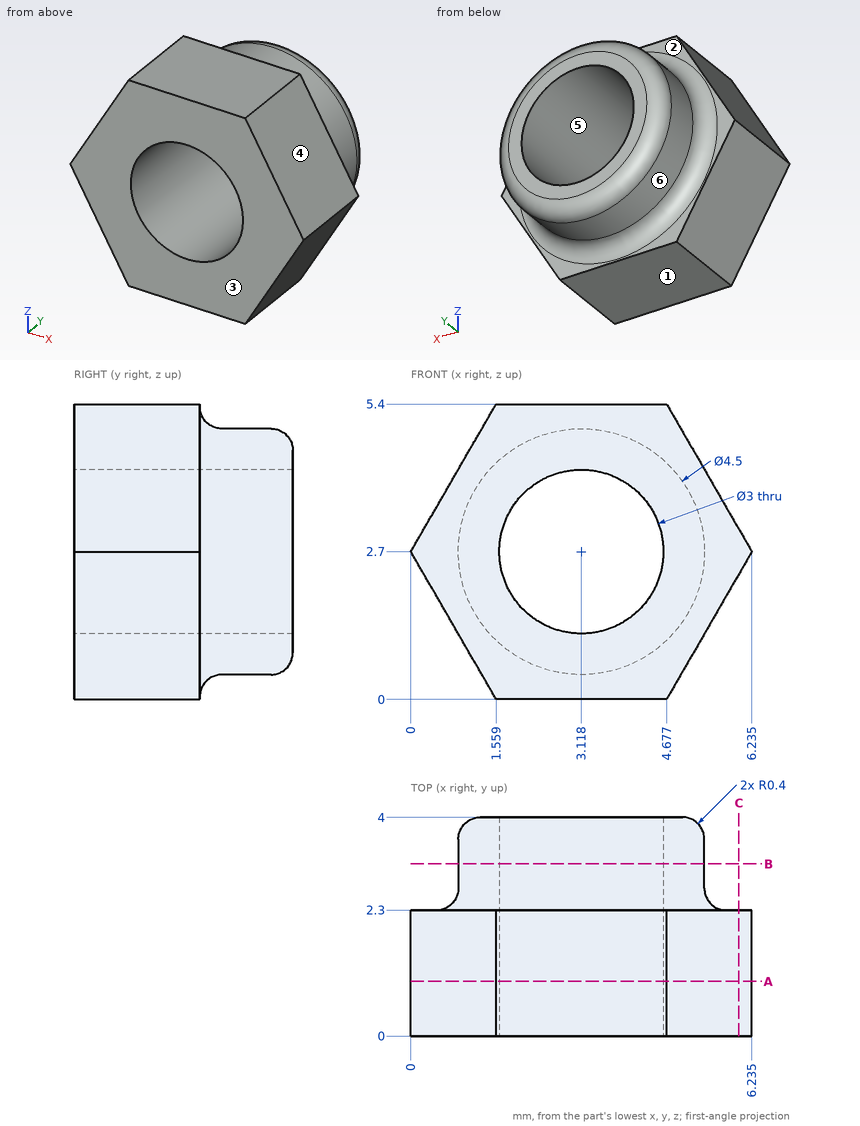
Geometry check sheet. Reference: drawing and pictorial views, mm from the part's lowest x, y, z. A direction names the side the tool comes from. Round coordinates to 2 decimals unless told otherwise and drop trailing zeros. Loops run counter-clockwise (first coordinate to the right, second up) from the corner with the lowest first, then second, coordinate; pieces in that order, holes last. Notation, with made-up numbers: (18.25, 30.5) - (71.25, 30.5) arc R28 ccw to (71.25, 67.5) - close; hole circle Ø5 at (20, 49). An arc over 180 degrees is marked (long way). Answer in a Markdown table with one row per item. Add a question column.
Q1. Gauge pin test, flat end, axial feed: pin 1 (1 mm diameter, centred on x = 2, y = 2, fed in from -Z). Record the tip position at first contact, or that the pin passes through.
Q2. Release check for a two-part mould opening along Z. For the marked faces 3, 4, 5 and 6 record: pulls with the +Z half, pulls with the -Z half, needs draft (parallel to the pull), parting line crosses it, or undercut.
Q3. Section check C-C on x = 6. Enter the section's corners in (y, z).
Q4. Tool access check on the marked faces 1 and 2. Record the directions out of +Z, -Z, +X, -X, +Y, -Y that give a thin tool (end or side, any length) a straight path to the whole face; none if there is none.
Q5. Material ranges on line 1 (X direction, y = 2.8, z = 2.7); line 2 (X direction, y = 3.55, z = 3.1) (1 decimal); line 3 (Z direction, x = 3.75, y = 3.05), recorded low to high.
Q6. Section check B-B on y = 3.15. Enter the section's corners in (x, z).
Q7. Section check A-A on y = 1. Enter the section's corners in (x, z) (1 decimal), plus the area to 3 significant figures.
Found:
| question | item | result |
|---|---|---|
| 1 | pin 1 | stops at z = 0 |
| 2 | face 3 | needs draft |
| 2 | face 4 | pulls with the +Z half |
| 2 | face 5 | undercut |
| 2 | face 6 | parting line crosses it |
| 3 | outline | (0, 2.29) - (2.3, 2.29) - (2.3, 3.11) - (0, 3.11) - close |
| 4 | face 1 | -Z, +X, -X, +Y, -Y |
| 4 | face 2 | +Y |
| 5 | line 1 | x = 0.87 to 1.62, 4.62 to 5.37 |
| 5 | line 2 | x = 0.9 to 1.7, 4.6 to 5.3 |
| 5 | line 3 | z = 0.54 to 1.34, 4.06 to 4.86 |
| 6 | outline | circle Ø4.5 at (3.12, 2.7); hole circle Ø3 at (3.12, 2.7) |
| 7 | outline | (0, 2.7) - (1.6, 0) - (4.7, 0) - (6.2, 2.7) - (4.7, 5.4) - (1.6, 5.4) - close; hole circle Ø3 at (3.1, 2.7) |
| 7 | area | 18.2 mm² |
